```python
from build123d import *

# Parameters (mm, degrees)
ESBO_O1_R                = 4
RESSALTO_EXTRUS_O1_DEPTH = 3
ESBO_O2_R                = 3
CORTE_EXTRUS_O1_DEPTH    = 2
ESBO_O3_R                = 2.5
RESSALTO_EXTRUS_O2_DEPTH = 1
ESBO_O4_R                = 1
CORTE_EXTRUS_O2_DEPTH    = 7.92820323


with BuildPart() as part:
    # Esboço1 → Ressalto-extrusão1 (new body)
    with BuildSketch(Plane(origin=(0, 0, 0), x_dir=(0, 0, -1), z_dir=(1, 0, 0))):
        Circle(ESBO_O1_R)
    extrude(amount=RESSALTO_EXTRUS_O1_DEPTH)

    # Esboço2 → Corte-extrusão1 (cut)
    with BuildSketch(Plane(origin=(3, 0, 0), x_dir=(0, 0, -1), z_dir=(1, 0, 0))):
        Circle(ESBO_O2_R)
    extrude(amount=-CORTE_EXTRUS_O1_DEPTH, mode=Mode.SUBTRACT)

    # Esboço3 → Ressalto-extrusão2 (add)
    with BuildSketch(Plane.ZY):
        Circle(ESBO_O3_R)
    extrude(amount=RESSALTO_EXTRUS_O2_DEPTH)

    # Esboço4 → Corte-extrusão2 (cut, through all)
    with BuildSketch(Plane.ZY.offset(1)):
        Circle(ESBO_O4_R)
    extrude(amount=-CORTE_EXTRUS_O2_DEPTH, mode=Mode.SUBTRACT)


solid = part.part
```
Read the model definition and answer for the solid it produces. Units are mm, in the model's axes. A direction names the side the tool comes from. Give positions to 0.01 mm unless a question says otherwise; leave off trailing zeros. Loops run counter-clockwise (first coordinate to the right, second up) from the corner with the lowest first, then second, coordinate; pieces in that order, holes last.
Item 1: For faces 1 (the cylindrical face through (2, 0, 3)), 2 (the cylindrical face through (-0.49, -2.44, -0.54)), 3 (the flat face through (-1, -1, 1)), determine the directions among +Z, -Z, +X, -X, +Y, -Y from which every point of the face is accessible in a straight line to the end or side of a thin tool.
Item 2: The part is cut by section D-D (y = -2.75). Write down the section's boundary in (x, z).
Item 3: The mould has two halves that part along Y. Classify faces 4 (the flat face through (3, 3, -1)), 5 (the cylindrical face through (1.479, -3.905, 0.867)), 6 (the cylindrical face through (0, -1, 0)): released by +Y, released by -Y, zero draft, split by the parting line, or undercut.
Item 4: The part is cut by section A-A (y = 0). Write down the section's boundary in (x, z).
Item 5: Find the intervals of material crossed by line 1 along Y through (x, z) = (0.2, 0); line 2 along Y through (x, z) = (1.9, 0); line 3 along X through (y, z) = (1.5, 0.25), in increasing order.
Item 6: The part is cut by section C-C (x = 2.65). Write down the section's boundary in (y, z).
Taken from the geometry:
1. face 1: +X
1. face 2: -X
1. face 3: +Z, -Z, -X, +Y, -Y
2. outline: (0, -2.9) - (3, -2.9) - (3, -1.2) - (1, -1.2) - (1, 1.2) - (3, 1.2) - (3, 2.9) - (0, 2.9) - close
3. face 4: zero draft
3. face 5: split by the parting line
3. face 6: undercut
4. outline: (-1, -2.5) - (0, -2.5) - (0, -4) - (3, -4) - (3, -3) - (1, -3) - (1, -1) - (-1, -1) - close; (-1, 1) - (1, 1) - (1, 3) - (3, 3) - (3, 4) - (0, 4) - (0, 2.5) - (-1, 2.5) - close
5. line 1: y = -4 to -1, 1 to 4
5. line 2: y = -4 to -3, 3 to 4
5. line 3: x = -1 to 1
6. outline: circle Ø8 at (0, 0); hole circle Ø6 at (0, 0)
